from build123d import *

# Parameters (mm, degrees)
BASEPLATE_W         = 105.3
BASEPLATE_H         = 105.3
BOSS_EXTRUDE1_DEPTH = 4
STANDS_R            = 5
STANDS_R_2          = 5.479963535
BOSS_EXTRUDE3_DEPTH = 2
CUT_EXTRUDE1_REACH  = 151.038
MOUNTING_HOLES_R    = 2.65
EDGE_CUTOUT_W       = 105.3
EDGE_CUTOUT_H       = 105.3
EDGE_CUTOUT_W_2     = 102.4
EDGE_CUTOUT_H_2     = 102.4
CUT_EXTRUDE2_DEPTH  = 1
FILLET_EDGES_R      = 8


with BuildPart() as part:
    # Baseplate → Boss-Extrude1 (new body)
    with BuildSketch(Plane(origin=(0, 0, 0), x_dir=(1, 0, 0), z_dir=(0, 1, 0))):
        with Locations((52.65, -52.65)):
            Rectangle(BASEPLATE_W, BASEPLATE_H)
    extrude(amount=BOSS_EXTRUDE1_DEPTH)

    # Stands → Boss-Extrude3 (add)
    with BuildSketch(Plane(origin=(0, 4, 0), x_dir=(1, 0, 0), z_dir=(0, 1, 0))):
        with Locations(Location((10.65, -10.65, 0), (0, 0, 270))):
            Circle(STANDS_R)
        with Locations(Location((94.65, -10.65, 0), (0, 0, 270))):
            Circle(STANDS_R_2)
        with Locations(Location((10.65, -94.65, 0), (0, 0, 270))):
            Circle(STANDS_R)
        with Locations(Location((94.65, -94.65, 0), (0, 0, 270))):
            Circle(STANDS_R)
    extrude(amount=BOSS_EXTRUDE3_DEPTH)

    # Mounting_Holes → Cut-Extrude1 (cut, up to next)
    with BuildSketch(Plane(origin=(0, 6, 0), x_dir=(1, 0, 0), z_dir=(0, 1, 0)), mode=Mode.PRIVATE) as cut_extrude1_sk1:
        with Locations(Location((10.65, -10.65, 0), (0, 0, 270))):
            Circle(MOUNTING_HOLES_R)
    cut_extrude1_tool1 = extrude(cut_extrude1_sk1.sketch, amount=-CUT_EXTRUDE1_REACH, mode=Mode.PRIVATE) & part.part
    # Mounting_Holes → Cut-Extrude1 (cut, up to next)
    with BuildSketch(Plane(origin=(0, 6, 0), x_dir=(1, 0, 0), z_dir=(0, 1, 0)), mode=Mode.PRIVATE) as cut_extrude1_sk2:
        with Locations(Location((94.65, -10.65, 0), (0, 0, 270))):
            Circle(MOUNTING_HOLES_R)
    cut_extrude1_tool2 = extrude(cut_extrude1_sk2.sketch, amount=-CUT_EXTRUDE1_REACH, mode=Mode.PRIVATE) & part.part
    # Mounting_Holes → Cut-Extrude1 (cut, up to next)
    with BuildSketch(Plane(origin=(0, 6, 0), x_dir=(1, 0, 0), z_dir=(0, 1, 0)), mode=Mode.PRIVATE) as cut_extrude1_sk3:
        with Locations(Location((94.65, -94.65, 0), (0, 0, 270))):
            Circle(MOUNTING_HOLES_R)
    cut_extrude1_tool3 = extrude(cut_extrude1_sk3.sketch, amount=-CUT_EXTRUDE1_REACH, mode=Mode.PRIVATE) & part.part
    # Mounting_Holes → Cut-Extrude1 (cut, up to next)
    with BuildSketch(Plane(origin=(0, 6, 0), x_dir=(1, 0, 0), z_dir=(0, 1, 0)), mode=Mode.PRIVATE) as cut_extrude1_sk4:
        with Locations(Location((10.65, -94.65, 0), (0, 0, 270))):
            Circle(MOUNTING_HOLES_R)
    cut_extrude1_tool4 = extrude(cut_extrude1_sk4.sketch, amount=-CUT_EXTRUDE1_REACH, mode=Mode.PRIVATE) & part.part
    add(cut_extrude1_tool1.solids().sort_by_distance((10.65, 6, 10.65))[0], mode=Mode.SUBTRACT)
    add(cut_extrude1_tool2.solids().sort_by_distance((94.65, 6, 10.65))[0], mode=Mode.SUBTRACT)
    add(cut_extrude1_tool3.solids().sort_by_distance((94.65, 6, 94.65))[0], mode=Mode.SUBTRACT)
    add(cut_extrude1_tool4.solids().sort_by_distance((10.65, 6, 94.65))[0], mode=Mode.SUBTRACT)

    # Edge_Cutout → Cut-Extrude2 (cut)
    with BuildSketch(Plane(origin=(0, 4, 0), x_dir=(1, 0, 0), z_dir=(0, 1, 0))):
        with Locations((52.65, -52.65)):
            Rectangle(EDGE_CUTOUT_W, EDGE_CUTOUT_H)
        with Locations((52.65, -52.65)):
            Rectangle(EDGE_CUTOUT_W_2, EDGE_CUTOUT_H_2, mode=Mode.SUBTRACT)
    extrude(amount=-CUT_EXTRUDE2_DEPTH, mode=Mode.SUBTRACT)

    # Fillet_Edges
    fillet_edges_edges = [part.edges().sort_by_distance(p)[0] for p in [
        (0, 1.5, 0),
        (105.3, 1.5, 0),
        (105.3, 1.5, 105.3),
        (0, 1.5, 105.3),
        (1.45, 3.5, 1.45),
        (103.85, 3.5, 1.45),
        (103.85, 3.5, 103.85),
        (1.45, 3.5, 103.85),
    ]]
    fillet(fillet_edges_edges, radius=FILLET_EDGES_R)


solid = part.part
Verification items for the finished model (mm, model axes). A direction names the side the tool comes from. Coordinates: 2 decimals unless noted, no trailing zeros. Order: outer loops, then holes, each group sorted by start corner. A loop starts at its lowest first (then second) coordinate and runs counter-clockwise, first axis right, second up. Notation, with made-up numbers: (-38, 31.5) -> (-6, 31.5) arc R10 ccw to (-6, 38.5) -> close; hole circle Ø11 at (66, 72.5). An arc over 180 degrees is marked (long way). Put each result on its own line as item: value. Start each with the question number.
1. Cross-section at A-A, the plane x = 94.65. Record the boundary of the cut face in (y, z).
2. Access from +Z, -Z, +X, -X, +Y, -Y to the whole of each face (thin tool, end or side, straight path). Record for faces 1 (the cylindrical face through (101.569, 3.493, 3.856)), 2 (the cylindrical face through (3.856, 3.493, 3.731)), 3 (the cylindrical face through (2.281, 1.521, 2.406)), 4 (the cylindrical face through (10.87, 4.986, 89.655)).
3. Cross-section at B-B, the plane z = 10.65. Record the boundary of the cut face in (x, y).
4. Cross-section at D-D, the plane z = 58. Record the boundary of the cut face in (x, y).
5. Mould release check, pull along Z, two halves, no side actions. Record for faces 5 (the cylindrical face through (101.444, 3.493, 101.569)), 6 (the flat face through (92, 6, 97)), 7 (the cylindrical face through (89.3, 4.99, 9.46)), 8 (the cylindrical face through (94.87, 4.986, 89.655)): released by +Z, released by -Z, zero draft, split by the parting line, or undercut.
6. Material ranges on L1, parallel to X at y = 2.05, z = 94.65; L2, parallel to X at y = 3.25, z = 94.65; L3, parallel to X at y = 4.05, z = 10.65, recorded low to high. Write a range as [from, to].
7. Cross-section at C-C, the plane x = 40. Record the boundary of the cut face in (y, z), then the cut area to 3 significant figures.
8. Go/stop test with flat-tipped pins: pin 1 Ø5 at (x, z) = (79, 41.5) entering from +Y; pin 2 Ø3 at (y, z) = (5, 93.5) entering from -X; pin 3 Ø4 at (x, z) = (10.65, 94.65) entering from +Y; pin 4 Ø0.5 at (x, y) = (68, 3.5) entering from -Z. Record where each tip stops, or that it passes through.
Computed:
1. outline: (0, 0) -> (3, 0) -> (3, 1.45) -> (4, 1.45) -> (4, 5.17) -> (6, 5.17) -> (6, 8) -> (0, 8) -> close; (0, 13.3) -> (6, 13.3) -> (6, 16.13) -> (4, 16.13) -> (4, 89.65) -> (6, 89.65) -> (6, 92) -> (0, 92) -> close; (0, 97.3) -> (6, 97.3) -> (6, 99.65) -> (4, 99.65) -> (4, 103.85) -> (3, 103.85) -> (3, 105.3) -> (0, 105.3) -> close
2. face 1: -Z, +X, +Y
2. face 2: -Z, -X, +Y
2. face 3: -Z, -X, +Y, -Y
2. face 4: +Y
3. outline: (0, 0) -> (8, 0) -> (8, 6) -> (5.65, 6) -> (5.65, 4) -> (1.45, 4) -> (1.45, 3) -> (0, 3) -> close; (13.3, 0) -> (92, 0) -> (92, 6) -> (89.17, 6) -> (89.17, 4) -> (15.65, 4) -> (15.65, 6) -> (13.3, 6) -> close; (97.3, 0) -> (105.3, 0) -> (105.3, 3) -> (103.85, 3) -> (103.85, 4) -> (100.13, 4) -> (100.13, 6) -> (97.3, 6) -> close
4. outline: (0, 0) -> (105.3, 0) -> (105.3, 3) -> (103.85, 3) -> (103.85, 4) -> (1.45, 4) -> (1.45, 3) -> (0, 3) -> close
5. face 5: released by +Z
5. face 6: zero draft
5. face 7: undercut
5. face 8: undercut
6. L1: [0, 8], [13.3, 92], [97.3, 105.3]
6. L2: [1.45, 8], [13.3, 92], [97.3, 103.85]
6. L3: [5.65, 8], [13.3, 15.65], [89.17, 92], [97.3, 100.13]
7. outline: (0, 0) -> (3, 0) -> (3, 1.45) -> (4, 1.45) -> (4, 103.85) -> (3, 103.85) -> (3, 105.3) -> (0, 105.3) -> close
7. area: 418 mm2
8. pin 1: y = 4
8. pin 2: x = 1.45
8. pin 3: through
8. pin 4: z = 1.45
